Geometry: see drawing. Coordinates: mm, zero at the bounding-box minimum. A direction names the side the tool comes from. Coordinates: 2 decimals unless noted, no trailing zeros. Loops run counter-clockwise (first coordinate to the right, second up) from the corner with the lowest first, then second, coordinate; pieces in that order, holes last. Notation, with made-up numbers: (2, 54) - (19, 54) arc R17 ccw to (19, 82) - close; hole circle Ø4 at (53.5, 44.25). An arc over 180 degrees is marked (long way). Write each question's results on one line, items separated by ' | '. Start each with the question number.
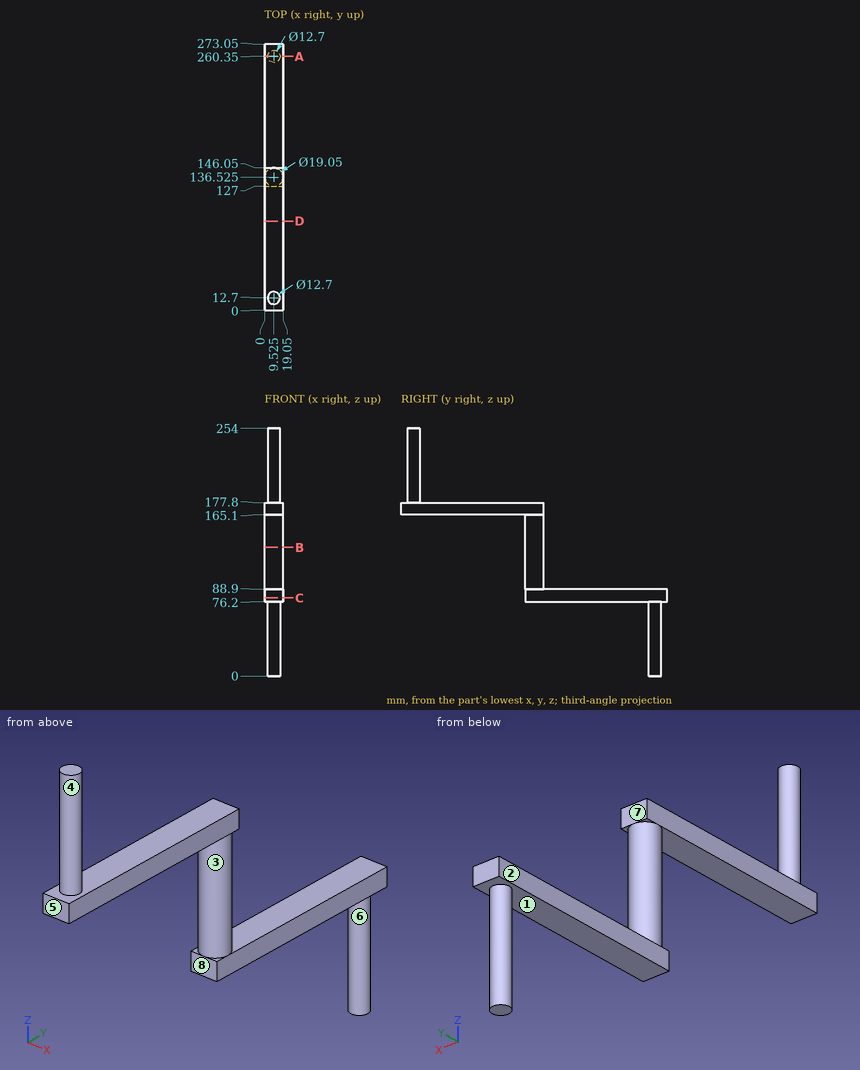
1) Section query B-B on z = 132. Output: boundary loops of the cut face in (x, y) (3 decimals).
2) Access query for the marked faces 4, 5, 6, 7 and 8. Directions: +Z, -Z, +X, -X, +Y, -Y. A direction counts if a zero-diameter tool reaches every point of the face in a straight line with its end or side. Return the directions, or none.
3) Section query D-D on y = 91.5. Output: boundary loops of the cut face in (x, z).
4) Pull-direction query (Z, two-part tool) for the marked faces 1, 2 and 3; classes: released by +Z, released by -Z, zero draft, split by the parting line, or undercut.
5) Pin query (flat end, axial travel): pin 1 Ø7.5 at (x, y) = (13, 129.5) entering from +Z; pin 2 Ø10 at (x, y) = (6, 66.5) entering from -Z; pin 3 Ø10.5 at (x, y) = (16, 140) entering from -Z. Return the tip coordinate at first contact, or that it passes through.
6) Material intervals for line 1 (Z direction, x = 18, y = 87); line 2 (Z direction, x = 11.5, y = 246); line 3 (Y direction, x = 4.25, z = 234.5), sorted ascending. Write a range as [from, to].
7) Section query C-C on z = 80. Output: boundary loops of the cut face in (x, y), and give its area (3 significant figures).
8) Section query A-A on y = 260.35. Output: boundary loops of the cut face in (x, z) (3 decimals).
Returned:
1) outline: circle Ø19.05 at (9.525, 136.525)
2) face 4: +Z | face 5: +Z, -Z, +X, -X, -Y | face 6: -Z | face 7: +Z, +X, -X, +Y | face 8: -Z, +X, -X, -Y
3) outline: (0, 165.1) - (19.05, 165.1) - (19.05, 177.8) - (0, 177.8) - close
4) face 1: released by -Z | face 2: zero draft | face 3: undercut
5) pin 1: stops at z = 177.8 | pin 2: stops at z = 165.1 | pin 3: stops at z = 76.2
6) line 1: z = [165.1, 177.8] | line 2: z = [76.2, 88.9] | line 3: y = [9.16, 16.24]
7) outline: (0, 127) - (19.05, 127) - (19.05, 273.05) - (0, 273.05) - close | area: 2,780 mm²
8) outline: (0, 76.2) - (3.175, 76.2) - (3.175, 0) - (15.875, 0) - (15.875, 76.2) - (19.05, 76.2) - (19.05, 88.9) - (0, 88.9) - close
